Autodesk Inventor part; units mm, degrees
ref_plane "Work Plane1" through (104.775, 0, 0) normal (0, 0, -1) x (1, 0, 0)
ref_plane "YZ Plane" through (0, 0, 0) normal (1, 0, 0) x (0, 1, 0)
ref_plane "XZ Plane" through (0, 0, 0) normal (0, 1, 0) x (-1, 0, 0)
sketch "Sketch1" plane through (0, 0, 0) normal (0, 0, 1) x (1, 0, 0)
  line L0 (12.7, 0) -> (12.7, 2.0828)
  line L1 (12.7, 2.0828) -> (4.8293, 2.0828)
  line L2 (4.8293, 2.0828) -> (2.8448, 2.0828)
  line L3 (0, 3.9497) -> (0, 1.3785)
  line L4 (0, 1.3785) -> (1.9304, 1.3785)
  line L5 (1.9304, 1.3785) -> (2.7263, 0)
  line L6 (2.7263, 0) -> (12.7, 0)
  line L7 (0, 3.9497) -> (0.6972, 3.9497)
  line L8 (0.6972, 3.9497) -> (2.8448, 2.0828)
  line L9 (2.8448, 2.0828) -> (2.8448, 2.0828)
  line L10 (4.8293, 2.0828) -> (2.8448, 2.0828) construction
  line L11 (2.8448, 2.0828) -> (2.8448, 2.0828)
  line L12 (-2.54, 0) -> (15.24, 0)
  line L13 (0, -0.7899) -> (0, 4.7396)
  dimension "d0" = 12.7
  dimension "d1" = 7.8707
  dimension "d2" = 1.9304
  dimension "d3" = 4.1656
  dimension "d6" = 2.8448
  dimension "d7" = 41
  dimension "d8" = 2.757
  dimension "d9" = 60
  dimension "d10" = 7.8994
  dimension "d11" = 4.1656
  dimension "d12" = 1.9845
revolve "Body" add sketch "Sketch1" angle 360 about axis through (2.7263, 0, 0) along (1, 0, 0) contours L6 L5 L4 L3 L7 L8 L2 L1 L0
sketch "Sketch2" plane through (0, 0, 0) normal (-1, 0, 0) x (0, 0, 1)
  circle A0 centre (0, 0) radius 1.3785
  line L0 (0, -5.5296) -> (0, 5.5296)
  line L1 (-5.5296, 0) -> (5.5296, 0)
  line L2 (1.3785, 0) -> (0.6892, -1.1938)
  line L3 (0.6892, -1.1938) -> (-0.6892, -1.1938)
  line L4 (-0.6892, -1.1938) -> (-1.3785, 0)
  line L5 (-1.3785, 0) -> (-0.6892, 1.1938)
  line L6 (-0.6892, 1.1938) -> (0.6892, 1.1938)
  line L7 (0.6892, 1.1938) -> (1.3785, 0)
  point P0 (0, 1.3785)
extrude "Slot" add sketch "Sketch2" against normal up to next contours L7 A0 | A0 L2 | L6 L0 A0 | A0 L0 L3 | L0 L6 A0 | A0 L3 L0 | L4 A0 | A0 L5
thread "Thread"
chamfer "Chamfer1" distance 0.4724 distance2 0.9449 1 edges at (12.7, -2.0828, 0) measured on face at (12.7, -0.7994, 0.0552)
ref_plane "Work Plane1" through (104.775, 0, 0) normal (0, 0, -1) x (1, 0, 0)
equation "\"d15\" = GEL"
equation "\"d17\" = -0.5 * SPD + 0.5 * GD"
equation "\"d18\" = GUL"
equation "\"d0\" = NLG"
equation "\"d1\" = GEL"
equation "\"d2\" = INTI"
equation "\"d3\" = GD"
equation "\"d6\" = KOH"
equation "\"d7\" = 0.5 * SEWI"
equation "\"d8\" = 1.1547 * SW"
equation "\"d10\" = KOD"
equation "\"d11\" = BDM"
equation "\"d12\" = GAL"
equation "\"NLG\" = 12.7"
equation "\"INTI\" = 1.9304"
equation "\"GEL\" = 7.8707"
equation "\"GAL\" = 1.9845"
equation "\"KOH\" = 2.8448"
equation "\"KOD\" = 7.8994"
equation "\"GUL\" = 0.94488"
equation "\"SPD\" = 3.22072"
equation "\"BDM\" = NND"
equation "\"GD\" = NND"
equation "\"SEWI\" = 82deg"
equation "\"SW\" = 2.3876"
equation "\"TOA\" = 30deg"
equation "\"GD1\" = SPD"
equation "\"THREADDIA\" = 4.1656"
equation "\"HHPTC\" = 0.79375"
equation "\"NND\" = 4.1656"
equation "\"E0\" = 1.155 * SW"
properties part number "ANSI B18.3 - 8-32 UNC x 0.5" material "Steel, Mild"
Source: CAD feature listing. Evaluate the final solid. Frame: model axes, mm. A direction names the side the tool comes from. Give positions to 0.01 mm unless a question says otherwise; leave off trailing zeros. Order: outer loops, then holes, each group sorted by start corner. A loop starts at its lowest first (then second) coordinate and runs counter-clockwise, first axis right, second up.
(1) Contact query for flat-ended pins moving along their axis: P1, Ø2, axis at x = 8.5, y = -2.5, coming from the -Z side (3 decimals); P2, Ø3, axis at x = 9, y = 1.5, coming from the +Z side; P3, Ø1, axis at x = 10, y = -1.5, coming from the +Z side; P4, Ø1, axis at y = 3, z = 1, coming from the -X side. Output: stop coordinate, or through.
(2) Section query B-B (x = 2.5). Return the cut outline in (y, z).
(3) Material intervals for line 1 along Z through (x, y) = (6.5, 0); line 2 along Z through (x, y) = (5.75, 1.25); line 3 along X through (y, z) = (3.5, -1.5), sorted ascending.
(4) Pull-direction query (Y, two-part tool) for faces 1 (the face through (0.353, -3.946, 0.174)), 2 (the face through (12.7, 0, 0)), 3 (the face through (1, 1.194, 0)); classes: +Y half, -Y half, draft (parallel to the pull), parting line (faces both ways), or undercut.
(5) Section query A-A (x = 9). Return the cut outline in (y, z).
(6) Access query for faces 4 (the face through (0, -1, -1)), 5 (the face through (7.238, 1.987, -0.626)), 6 (the face through (1.004, -0.605, -1.029)). Directions: +Z, -Z, +X, -X, +Y, -Y. A direction counts if a zero-diameter tool reaches every point of the face in a straight line with its end or side. Return the directions, or none.
Outcome:
1. P1: stops at z = -1.445
1. P2: stops at z = 2.08
1. P3: stops at z = 1.83
1. P4: stops at x = 0
2. outline: circle Ø4.77 at (0, 0); hole circle Ø0.78 at (0, 0)
3. line 1: z = -2.08 to 2.08
3. line 2: z = -1.67 to 1.67
3. line 3: x = 0 to 0.86
4. face 1: parting line
4. face 2: draft
4. face 3: undercut
5. outline: circle Ø4.17 at (0, 0)
6. face 4: +Z, -Z, -X, +Y, -Y
6. face 5: +X
6. face 6: -X
